Can you work these out from the drawing? Everything is in mm from the part's minimum corner. Round coordinates to 2 decimals unless told otherwise and drop trailing zeros. Order: outer loops, then holes, each group sorted by start corner. A loop starts at its lowest first (then second) coordinate and runs counter-clockwise, first axis right, second up. Notation, with made-up numbers: (58.25, -11) -> (67.25, -11) arc R35 ccw to (67.25, 28) -> close; hole circle Ø3 at (-15, -15). An arc over 180 degrees is marked (long way). One line per item, written item: value.
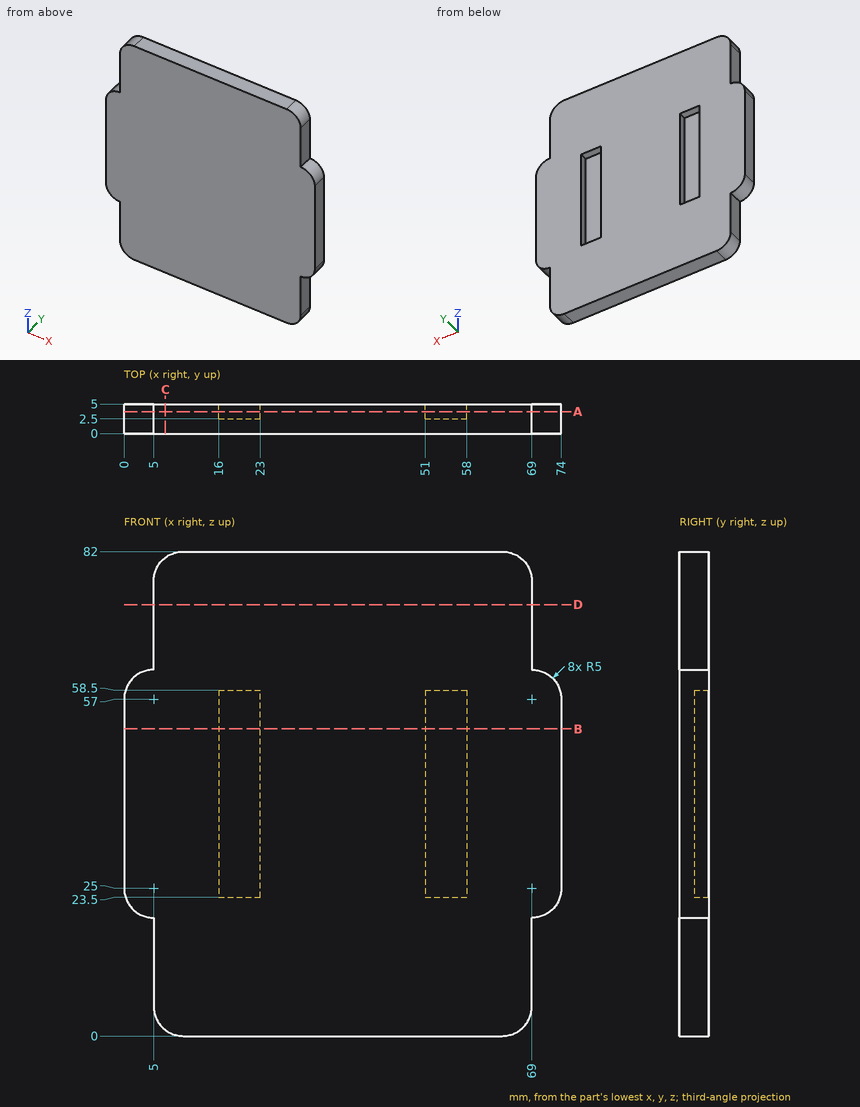
Q1. Please list where these lines run through material, in increasing order: line 1 along X through (y, z) = (2.65, 24); line 2 along X through (y, z) = (3.85, 66); line 3 along Y through (x, z) = (21.5, 32).
Answers below:
line 1: 0.1 to 16, 23 to 51, 58 to 73.9
line 2: 5 to 69
line 3: 0 to 2.5
Q2. I want a section at B-B on z = 52. List the corners of the cut face in (x, y) for me, plus the area to 3 significant figures.
Answers below:
outline: (0, 0) -> (74, 0) -> (74, 5) -> (58, 5) -> (58, 2.5) -> (51, 2.5) -> (51, 5) -> (23, 5) -> (23, 2.5) -> (16, 2.5) -> (16, 5) -> (0, 5) -> close
area: 335 mm^2
Q3. I want a section at D-D on z = 73. List the corners of the cut face in (x, y) for me, plus the area to 3 significant figures.
Answers below:
outline: (5, 0) -> (69, 0) -> (69, 5) -> (5, 5) -> close
area: 320 mm^2
Q4. I want a section at C-C on x = 7. List the corners of the cut face in (y, z) for me, plus the area to 3 significant figures.
Answers below:
outline: (0, 1) -> (5, 1) -> (5, 81) -> (0, 81) -> close
area: 400 mm^2
Q5. I want a section at A-A on y = 3.7. List the corners of the cut face in (x, z) for me, plus the area to 3 significant figures.
Answers below:
outline: (0, 25) arc R5 ccw to (5, 20) -> (5, 5) arc R5 ccw to (10, 0) -> (64, 0) arc R5 ccw to (69, 5) -> (69, 20) arc R5 ccw to (74, 25) -> (74, 57) arc R5 ccw to (69, 62) -> (69, 77) arc R5 ccw to (64, 82) -> (10, 82) arc R5 ccw to (5, 77) -> (5, 62) arc R5 ccw to (0, 57) -> close; hole (16, 23.5) -> (23, 23.5) -> (23, 58.5) -> (16, 58.5) -> close; hole (51, 23.5) -> (58, 23.5) -> (58, 58.5) -> (51, 58.5) -> close
area: 5,140 mm^2
Q6. Will these pins go through, and if not, where does the flat tip stop? pin 1 Ø1.5 at (y, z) = (1.5, 15) entering from -X; pin 2 Ø3.5 at (x, z) = (18, 38) entering from +Y; pin 3 Ø1.5 at (y, z) = (3.5, 13.5) entering from +X.
Answers below:
pin 1: x = 5
pin 2: y = 2.5
pin 3: x = 69
